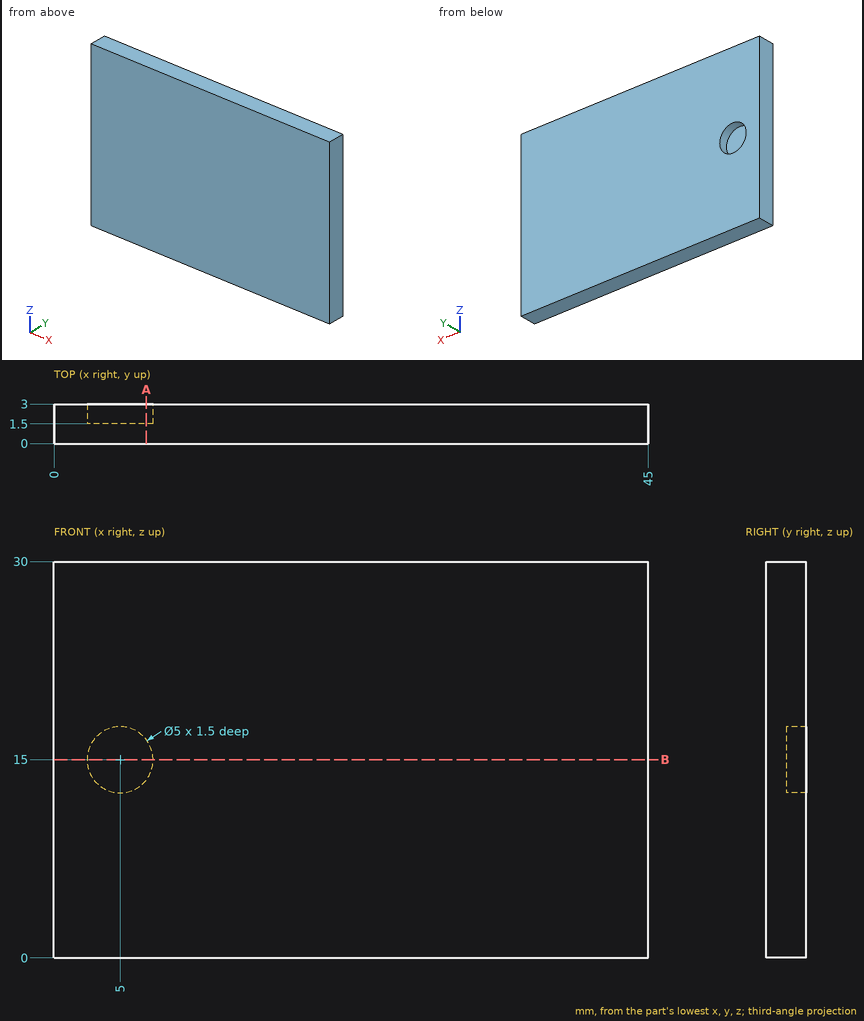
Answer from the drawing. Dimensions are ordinates in mm from the lowest x, y and z of the part. Round coordinates to 2 decimals unless told otherwise and drop trailing zeros. Order: outer loops, then holes, each group sorted by start corner. A loop starts at its lowest first (then second) coordinate and runs counter-clockwise, first axis right, second up. Notation, with made-up numbers: (67.25, 12) -> (72.25, 12) arc R11 ccw to (72.25, 22) -> close; hole circle Ø5 at (48.25, 54.25). An arc over 180 degrees is marked (long way). Answer as CSV lines item,"result".
Q1. Consider line 1 (Z direction, x = 5, y = 2.6); line 2 (Z direction, x = 3.5, y = 1.7). Determine where each line is inside the solid, lowest interval first. Write a range as from..to.
Computed values:
line 1,"z = 0..12.5, 17.5..30"
line 2,"z = 0..13, 17..30"
Q2. A cutting plane is placed at B-B on z = 15. Determine the outline of the cut face in (x, y), plus the area to 4 significant figures.
Computed values:
outline,"(0, 0) -> (45, 0) -> (45, 3) -> (7.5, 3) -> (7.5, 1.5) -> (2.5, 1.5) -> (2.5, 3) -> (0, 3) -> close"
area,"127.5 mm^2"
Q3. Given pin 1 (3 mm diameter, centred on x = 5, z = 15, fed in from -Y); pin 2 (1.5 mm diameter, centred on x = 4, z = 15, fed in from +Y), each flat-ended and moving along its own axis, determine where each tip first touches the part or whether it passes through.
Computed values:
pin 1,"stops at y = 0"
pin 2,"stops at y = 1.5"
Q4. A cutting plane is placed at A-A on x = 7. Determine the outline of the cut face in (y, z), plus the area to 3 significant figures.
Computed values:
outline,"(0, 0) -> (3, 0) -> (3, 13.5) -> (1.5, 13.5) -> (1.5, 16.5) -> (3, 16.5) -> (3, 30) -> (0, 30) -> close"
area,"85.5 mm^2"
